Can you work these out from the model? Positions are in its coordinate system, mm. A direction names the side the tool comes from. Round coordinates to 2 decimals unless told otherwise and drop trailing zeros. Loops run counter-clockwise (first coordinate to the right, second up) from the corner with the lowest first, then second, coordinate; pieces in that order, holes last. Notation, with made-up numbers: (53, -9) -> (62, -9) arc R7 ccw to (62, -4) -> close; hole circle Ø8 at (22, 51). An arc over 180 degrees is marked (long way). Answer as a JSON object with one key per item and string values.
```python
from build123d import *

# Parameters (mm, degrees)
SKETCH1_W                         = 3
SKETCH1_H                         = 68.094259971
MAIN_EXTRUDE_DEPTH                = 54.25
SKETCH2_W                         = 8
SKETCH2_H                         = 68.094259971
TOP_SCREWHOLE_EXTENSION_DEPTH     = 3
SKETCH3_W                         = 8
SKETCH3_H                         = 68.094259971
BOTTOM_SCREWHOLE_EXTENSION_DEPTH  = 3
SCREWHOLE_EXTENSION_FILLETS_5MM_R = 5
SKETCH4_R                         = 1.5
BOTTOM_SCREWHOLES_DEPTH           = 8
TOP_START                         = -8
SKETCH5_R                         = 1.5
TOP_SCREWHOLES_DEPTH              = 8
WEIGHT_REDUCTION_DEPTH            = 101.505676109
WEIGHT_REDUCTION_DEPTH_BACK       = 101.505676109


with BuildPart() as part:
    # Sketch1 → Main extrude (new body)
    with BuildSketch(Plane(origin=(0, -6.84807753, 0), x_dir=(1, 0, 0), z_dir=(0, 1, 0))):
        with Locations((97.25, 54.216388238)):
            Rectangle(SKETCH1_W, SKETCH1_H)
    extrude(amount=MAIN_EXTRUDE_DEPTH)

    # Sketch2 → Top screwhole extension (add)
    with BuildSketch(Plane(origin=(0, 47.40192247, 0), x_dir=(1, 0, 0), z_dir=(0, 1, 0))):
        with Locations((94.75, 54.216388238)):
            Rectangle(SKETCH2_W, SKETCH2_H)
    extrude(amount=-TOP_SCREWHOLE_EXTENSION_DEPTH)

    # Sketch3 → Bottom screwhole extension (add)
    with BuildSketch(Plane.XZ.offset(6.84807753)):
        with Locations((94.75, -54.216388238)):
            Rectangle(SKETCH3_W, SKETCH3_H)
    extrude(amount=-BOTTOM_SCREWHOLE_EXTENSION_DEPTH)

    # Screwhole extension fillets 5mm
    screwhole_extension_fillets_5mm_edges = [part.edges().sort_by_distance(p)[0] for p in [
        (95.75, 44.40192247, -54.216388238),
        (95.75, -3.84807753, -54.216388238),
    ]]
    fillet(screwhole_extension_fillets_5mm_edges, radius=SCREWHOLE_EXTENSION_FILLETS_5MM_R - 0.0001)  # a hair under: the kernel refuses the full size

    # Sketch4 → Bottom screwholes (cut)
    with BuildSketch(Plane.XZ.offset(6.84807753)):
        with Locations(Location((94.75, -25.169258252, 0), (0, 0, 270))):
            Circle(SKETCH4_R)
        with Locations(Location((94.75, -83.263518223, 0), (0, 0, 270))):
            Circle(SKETCH4_R)
    extrude(amount=-BOTTOM_SCREWHOLES_DEPTH, mode=Mode.SUBTRACT)

    # Sketch5 → Top screwholes (cut)
    with BuildSketch(Plane(origin=(0, 47.40192247, 0), x_dir=(1, 0, 0), z_dir=(0, 1, 0)).offset(TOP_START)):
        with Locations(Location((94.75, 25.169258252, 0), (0, 0, 90))):
            Circle(SKETCH5_R)
        with Locations(Location((94.75, 83.263518223, 0), (0, 0, 90))):
            Circle(SKETCH5_R)
    extrude(amount=TOP_SCREWHOLES_DEPTH, mode=Mode.SUBTRACT)

    # Sketch6 → Weight reduction (cut, two sides: drawn at the far end of the back side and taken through both)
    with BuildSketch(Plane(origin=(98.75, 0, 0), x_dir=(0, 0, -1), z_dir=(1, 0, 0)).offset(-WEIGHT_REDUCTION_DEPTH_BACK)):
        with BuildLine():
            Line((28.169258252, 34.40192247), (28.169258252, 6.15192247))
            ThreePointArc((28.169258252, 6.15192247), (29.633724346, 2.616388564), (33.169258252, 1.15192247))
            Line((33.169258252, 1.15192247), (75.263518223, 1.15192247))
            ThreePointArc((75.263518223, 1.15192247), (78.799052129, 2.616388564), (80.263518223, 6.15192247))
            Line((80.263518223, 6.15192247), (80.263518223, 34.40192247))
            ThreePointArc((80.263518223, 34.40192247), (78.799052129, 37.937456376), (75.263518223, 39.40192247))
            Line((75.263518223, 39.40192247), (33.169258252, 39.40192247))
            ThreePointArc((33.169258252, 39.40192247), (29.633724346, 37.937456376), (28.169258252, 34.40192247))
        make_face()
    extrude(amount=WEIGHT_REDUCTION_DEPTH + WEIGHT_REDUCTION_DEPTH_BACK, mode=Mode.SUBTRACT)


solid = part.part
```
Q1. I want a section at C-C, the plane x = 94. Write out the boundary of the cut face in (y, z), then the cut area to 3 significant figures.
Determined:
{"outline": "(-6.85, -88.26) -> (-2.65, -88.26) -> (-2.65, -84.56) -> (-6.85, -84.56) -> close; (-6.85, -81.96) -> (-2.65, -81.96) -> (-2.65, -26.47) -> (-6.85, -26.47) -> close; (-6.85, -23.87) -> (-2.65, -23.87) -> (-2.65, -20.17) -> (-6.85, -20.17) -> close; (43.2, -88.26) -> (47.4, -88.26) -> (47.4, -84.56) -> (43.2, -84.56) -> close; (43.2, -81.96) -> (47.4, -81.96) -> (47.4, -26.47) -> (43.2, -26.47) -> close; (43.2, -23.87) -> (47.4, -23.87) -> (47.4, -20.17) -> (43.2, -20.17) -> close", "area": "528 mm²"}
Q2. On a 3-axis mill with a long thin cutter (end or side, diameter ignored), from which of +Z, -Z, +X, -X, +Y, -Y can I reach the whole of each face in a straight line? I mean faces 5 (the cylindrical face through (96.237, -3.793, -83.068)), 6 (the flat face through (96, 20, -20.169)), 7 (the cylindrical face through (94.25, -2.42, -53.74)), 8 (the flat face through (97, 1.152, -54)), 9 (the cylindrical face through (96.214, 44.235, -24.844)). Say none if no direction works.
Determined:
{"face 5": "-Y", "face 6": "+Z, +X, -X, +Y, -Y", "face 7": "+Z, -Z, -X", "face 8": "+X, -X", "face 9": "+Y"}
Q3. We'd pull the mould along Y, two halves only. Please class faces 1 (the flat face through (95, -6.848, -54)), 2 (the flat face through (95.75, 20, -26)), 3 (the cylindrical face through (97.23, 2.58, -78.76)), 4 (the cylindrical face through (96.214, 44.235, -82.938)): pulls with the +Y half, pulls with the -Y half, needs draft (parallel to the pull), parting line crosses it, or undercut.
Determined:
{"face 1": "pulls with the -Y half", "face 2": "undercut", "face 3": "undercut", "face 4": "needs draft"}
Q4. I want a section at D-D, the plane y = 43.5. Write out the boundary of the cut face in (x, z).
Determined:
{"outline": "(93.61, -88.26) -> (98.75, -88.26) -> (98.75, -20.17) -> (93.61, -20.17) -> (93.61, -24.19) arc R1.5 cw (long way) to (93.61, -26.15) -> (93.61, -82.28) arc R1.5 cw (long way) to (93.61, -84.24) -> close"}
Q5. I'm going to push a flat-ended pin straight in: pin 1 (2.5 mm diameter, centred on x = 94.75, z = -83.26, fed in from +Y). Where does the tip first touch, or does it pass through?
Determined:
{"pin 1": "y = 39.4"}
Q6. I want a section at A-A, the plane y = 22.5. Write out the boundary of the cut face in (x, z), then the cut area to 3 significant figures.
Determined:
{"outline": "(95.75, -88.26) -> (98.75, -88.26) -> (98.75, -80.26) -> (95.75, -80.26) -> close; (95.75, -28.17) -> (98.75, -28.17) -> (98.75, -20.17) -> (95.75, -20.17) -> close", "area": "48.0 mm²"}
Q7. If I drill on L1, parallel to Z at x = 94.75, y = 42.75; L2, parallel to Z at x = 96.25, y = 33.5; L3, parallel to Y at x = 98, z = -59.5, over which ranges is the centre line in solid material (lowest first)? Write a range as [from, to].
Determined:
{"L1": "[-88.26, -84.76], [-81.76, -26.67], [-23.67, -20.17]", "L2": "[-88.26, -80.26], [-28.17, -20.17]", "L3": "[-6.85, 1.15], [39.4, 47.4]"}
